Design review of the part built by this model. Coordinates are the model's own, in mm. Round coordinates to 2 decimals unless told otherwise and drop trailing zeros. Order: outer loops, then holes, each group sorted by start corner. A loop starts at its lowest first (then second) coordinate and runs counter-clockwise, first axis right, second up. Notation, with made-up numbers: (-6, 60) - (40, 60) arc R37 cw to (40, 96) - close; hole circle Ø3 at (65.5, -15.75). An arc over 180 degrees is marked (long way). Write item = value, one per line.
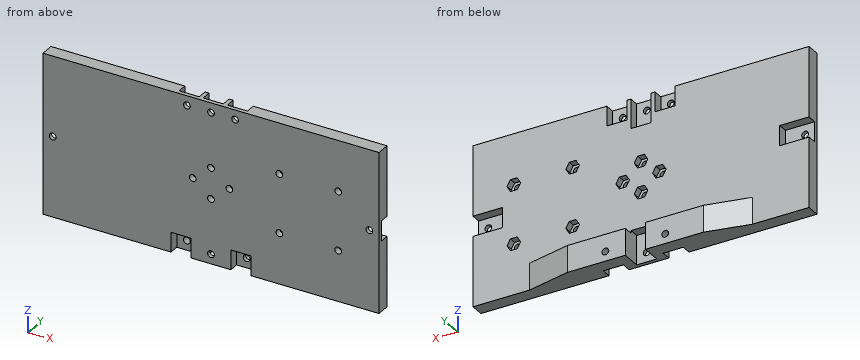
from build123d import *
from build123d.topology import SkipClean

# Parameters (mm, degrees)
SKETCH1_W           = 174.17
SKETCH1_H           = 83
BOSS_EXTRUDE1_DEPTH = 7
SKETCH2_R           = 1.75
CUT_EXTRUDE1_DEPTH  = 194.062655374
SKETCH3_R           = 1.75
CUT_EXTRUDE2_DEPTH  = 194.062655374
SKETCH4_W           = 15.4
SKETCH4_H           = 10.4
SKETCH4_W_2         = 10.4
SKETCH4_H_2         = 15.4
CUT_EXTRUDE3_DEPTH  = 5
SKETCH5_W           = 10.4
SKETCH5_H           = 10.4
CUT_EXTRUDE4_DEPTH  = 5
SKETCH6_R           = 1.75
CUT_EXTRUDE5_DEPTH  = 194.000489378
SKETCH12_R          = 1.75
CUT_EXTRUDE9_DEPTH  = 194.062655374
CUT_EXTRUDE6_DEPTH  = 3.64
SKETCH9_W           = 10.4
SKETCH9_H           = 10.4
CUT_EXTRUDE7_DEPTH  = 5
SKETCH10_R          = 1.75
CUT_EXTRUDE8_DEPTH  = 194.000489378
SKETCH13_W          = 20.6
SKETCH13_H          = 13.86
SKETCH13_R          = 1.75
BOSS_EXTRUDE2_DEPTH = 5
CHAMFER1_SIZE       = 7.094229205
CHAMFER1_SIZE_2     = 32
MIRROR1_START       = -76.250259333
MIRROR1_DEPTH       = 7.110259333
MIRROR1_START_2     = -83
MIRROR1_2_DEPTH     = 3.2499999
MIRROR1_START_3     = -79.7500001
MIRROR1_3_DEPTH     = 3.499740767
MIRROR1_START_4     = 7
MIRROR1_4_OUTLINE_R = 1.75
MIRROR1_4_DEPTH     = 5


with BuildPart() as part:
    # Sketch1 → Boss-Extrude1 (new body)
    with BuildSketch(Plane(origin=(0, 0, 0), x_dir=(1, 0, 0), z_dir=(0, 1, 0))):
        with Locations((87.085, 41.5)):
            Rectangle(SKETCH1_W, SKETCH1_H)
    extrude(amount=BOSS_EXTRUDE1_DEPTH)

    # Sketch2 → Cut-Extrude1 (cut, through all)
    with BuildSketch(Plane(origin=(0, 7, 0), x_dir=(1, 0, 0), z_dir=(0, 1, 0))):
        with Locations(Location((87.085, 49.5, 0), (0, 0, 270))):
            Circle(SKETCH2_R)
        with Locations(Location((77.585, 41.5, 0), (0, 0, 270))):
            Circle(SKETCH2_R)
        with Locations(Location((96.585, 41.5, 0), (0, 0, 270))):
            Circle(SKETCH2_R)
        with Locations(Location((87.085, 33.5, 0), (0, 0, 270))):
            Circle(SKETCH2_R)
    extrude(amount=-CUT_EXTRUDE1_DEPTH, mode=Mode.SUBTRACT)

    # Sketch3 → Cut-Extrude2 (cut, through all)
    with BuildSketch(Plane(origin=(0, 7, 0), x_dir=(1, 0, 0), z_dir=(0, 1, 0))):
        with Locations(Location((87.085, 78, 0), (0, 0, 270))):
            Circle(SKETCH3_R)
        with Locations(Location((5, 41.5, 0), (0, 0, 270))):
            Circle(SKETCH3_R)
        with Locations(Location((87.085, 5, 0), (0, 0, 270))):
            Circle(SKETCH3_R)
        with Locations(Location((169.17, 41.5, 0), (0, 0, 270))):
            Circle(SKETCH3_R)
    extrude(amount=-CUT_EXTRUDE2_DEPTH, mode=Mode.SUBTRACT)

    # Sketch4 → Cut-Extrude3 (cut)
    with BuildSketch(Plane(origin=(0, 7, 0), x_dir=(1, 0, 0), z_dir=(0, 1, 0))):
        with Locations((7.5, 41.5)):
            Rectangle(SKETCH4_W, SKETCH4_H)
        with Locations((87.085, 7.5)):
            Rectangle(SKETCH4_W_2, SKETCH4_H_2)
        with Locations((87.085, 75.5)):
            Rectangle(SKETCH4_W_2, SKETCH4_H_2)
        with Locations((166.67, 41.5)):
            Rectangle(SKETCH4_W, SKETCH4_H)
    extrude(amount=-CUT_EXTRUDE3_DEPTH, mode=Mode.SUBTRACT)

    # Sketch5 → Cut-Extrude4 (cut)
    with BuildSketch(Plane(origin=(0, 7, 0), x_dir=(1, 0, 0), z_dir=(0, 1, 0))):
        with Locations((74.585, 5)):
            Rectangle(SKETCH5_W, SKETCH5_H)
        with Locations((99.585, 5)):
            Rectangle(SKETCH5_W, SKETCH5_H)
    extrude(amount=-CUT_EXTRUDE4_DEPTH, mode=Mode.SUBTRACT)

    # Sketch6 → Cut-Extrude5 (cut, through all)
    with BuildSketch(Plane(origin=(0, 2, 0), x_dir=(1, 0, 0), z_dir=(0, 1, 0))):
        with Locations(Location((74.585, 5, 0), (0, 0, 270))):
            Circle(SKETCH6_R)
        with Locations(Location((99.585, 5, 0), (0, 0, 270))):
            Circle(SKETCH6_R)
    extrude(amount=-CUT_EXTRUDE5_DEPTH, mode=Mode.SUBTRACT)

    # Sketch12 → Cut-Extrude9 (cut, through all)
    with BuildSketch(Plane.XZ):
        with Locations(Location((122.51393219, -26.25, 0), (0, 0, 270))):
            Circle(SKETCH12_R)
        with Locations(Location((153.01393219, -26.25, 0), (0, 0, 270))):
            Circle(SKETCH12_R)
        with Locations(Location((122.51393219, -56.75, 0), (0, 0, 270))):
            Circle(SKETCH12_R)
        with Locations(Location((153.01393219, -56.75, 0), (0, 0, 270))):
            Circle(SKETCH12_R)
    extrude(amount=-CUT_EXTRUDE9_DEPTH, mode=Mode.SUBTRACT)

    # Sketch7 → Cut-Extrude6 (cut)
    with BuildSketch(Plane(origin=(0, 7, 0), x_dir=(1, 0, 0), z_dir=(0, 1, 0))):
        Polygon((75.824081679, 44.55), (79.345918321, 44.55), (81.106836642, 41.5), (79.345918321, 38.45), (75.824081679, 38.45), (74.063163358, 41.5), align=None)
        Polygon((85.324081679, 52.55), (88.845918321, 52.55), (90.606836642, 49.5), (88.845918321, 46.45), (85.324081679, 46.45), (83.563163358, 49.5), align=None)
        Polygon((100.106836642, 41.5), (98.345918321, 44.55), (94.824081679, 44.55), (93.063163358, 41.5), (94.824081679, 38.45), (98.345918321, 38.45), align=None)
        Polygon((83.563163358, 33.5), (85.324081679, 30.45), (88.845918321, 30.45), (90.606836642, 33.5), (88.845918321, 36.55), (85.324081679, 36.55), align=None)
        Polygon((120.753013869, 29.3), (124.274850511, 29.3), (126.035768832, 26.25), (124.274850511, 23.2), (120.753013869, 23.2), (118.992095548, 26.25), align=None)
        Polygon((151.253013869, 29.3), (154.774850511, 29.3), (156.535768832, 26.25), (154.774850511, 23.2), (151.253013869, 23.2), (149.492095548, 26.25), align=None)
        Polygon((151.253013869, 59.8), (154.774850511, 59.8), (156.535768832, 56.75), (154.774850511, 53.7), (151.253013869, 53.7), (149.492095548, 56.75), align=None)
        Polygon((120.753013869, 59.8), (124.274850511, 59.8), (126.035768832, 56.75), (124.274850511, 53.7), (120.753013869, 53.7), (118.992095548, 56.75), align=None)
    extrude(amount=-CUT_EXTRUDE6_DEPTH, mode=Mode.SUBTRACT)

    # Sketch9 → Cut-Extrude7 (cut)
    with BuildSketch(Plane.XZ):
        with Locations((71.585, -78)):
            Rectangle(SKETCH9_W, SKETCH9_H)
        with Locations((102.585, -78)):
            Rectangle(SKETCH9_W, SKETCH9_H)
    extrude(amount=-CUT_EXTRUDE7_DEPTH, mode=Mode.SUBTRACT)

    # Sketch10 → Cut-Extrude8 (cut, through all)
    with BuildSketch(Plane.XZ.offset(-5)):
        with Locations(Location((71.585, -78, 0), (0, 0, 270))):
            Circle(SKETCH10_R)
        with Locations(Location((102.585, -78, 0), (0, 0, 270))):
            Circle(SKETCH10_R)
    extrude(amount=-CUT_EXTRUDE8_DEPTH, mode=Mode.SUBTRACT)

    # Sketch13 → Boss-Extrude2 (add)
    with BuildSketch(Plane(origin=(0, 7, 0), x_dir=(1, 0, 0), z_dir=(0, 1, 0))):
        with Locations((71.585, 76.07)):
            Rectangle(SKETCH13_W, SKETCH13_H)
        with Locations(Location((71.585, 78, 0), (0, 0, 90))):
            Circle(SKETCH13_R, mode=Mode.SUBTRACT)
    extrude(amount=BOSS_EXTRUDE2_DEPTH)

    # Chamfer1
    # the kernel refuses this chamfer: 32, 7.094229205 mm, written as the material it adds along each edge
    with BuildSketch(Plane(origin=(61.285, 7, -83), x_dir=(0, 1, 0), z_dir=(0, 0, 1))) as chamfer1_piece_1_section:
        Polygon((CHAMFER1_SIZE, 0), (0, CHAMFER1_SIZE_2), (0, 0), align=None)
    chamfer1_piece_1 = extrude(amount=13.86, mode=Mode.PRIVATE)
    chamfer1_piece_1 = split(chamfer1_piece_1, bisect_by=Plane(origin=(61.285, 12, -83), z_dir=(0, -1, 0)), keep=Keep.TOP, mode=Mode.PRIVATE)
    add(chamfer1_piece_1)

    # Mirror1: read off the stored shape, not the designer's step
    # Mirror1 outline → Mirror1 (add)
    with BuildSketch(Plane.XY.offset(MIRROR1_START)):
        Polygon((92.285, 12), (92.285, 7), (144.885, 7), (122.331457482, 12), align=None)
    extrude(amount=MIRROR1_DEPTH)

    # Mirror1 2 outline → Mirror1 2 (add)
    with BuildSketch(Plane.XY.offset(MIRROR1_START_2)):
        Polygon((92.285, 12), (92.285, 7), (144.885, 7), (122.331457482, 12), align=None)
    extrude(amount=MIRROR1_2_DEPTH)

    # Mirror1 3 outline → Mirror1 3 (add)
    with BuildSketch(Plane.XY.offset(MIRROR1_START_3)):
        Polygon((92.285, 12), (92.285, 7), (144.885, 7), (122.331457482, 12), align=None)
    extrude(amount=MIRROR1_3_DEPTH)

    # Mirror1 4 outline → Mirror1 4 (cut)
    with SkipClean():  # the faces are left unmerged after this step: merging them gives an invalid solid
        with BuildSketch(Plane(origin=(0, 0, 0), x_dir=(1, 0, 0), z_dir=(0, 1, 0)).offset(MIRROR1_START_4)):
            with Locations((102.585, 78)):
                Circle(MIRROR1_4_OUTLINE_R)
        extrude(amount=MIRROR1_4_DEPTH, mode=Mode.SUBTRACT)
    add(part.part.scale(1), mode=Mode.REPLACE)  # the faces are merged on a copy


solid = part.part
Item 1: For line 1 along X through (y, z) = (1.05, -26.25); line 2 along Z through (x, y) = (164, 4); line 3 along X through (y, z) = (6.5, -43.5), list the stretches that pass through material, from the lowest coordinate up. Write a range as [from, to].
Data:
line_1 = [0, 120.76], [124.26, 151.26], [154.76, 174.17]
line_2 = [-83, -46.7], [-36.3, 0]
line_3 = [15.2, 75.22], [79.95, 94.22], [98.95, 158.97]
Item 2: Take a section at C-C, the plane x = 36. State the section outline as (y, z) points, and give its area (3 significant figures).
Data:
outline = (0, -83) - (8.49, -83) - (8.49, -69.14) - (7, -69.14) - (7, 0) - (0, 0) - close
area = 602 mm2
Item 3: Take a section at B-B, the plane z = -17. State the section outline as (x, y) points, and give its area (3 significant figures).
Data:
outline = (0, 0) - (174.17, 0) - (174.17, 7) - (0, 7) - close
area = 1,220 mm2
Item 4: Take a section at A-A, the plane x = 169.17. State the section outline as (y, z) points.
Data:
outline = (0, -83) - (7, -83) - (7, -46.7) - (2, -46.7) - (2, -43.25) - (0, -43.25) - close; (0, -39.75) - (2, -39.75) - (2, -36.3) - (7, -36.3) - (7, 0) - (0, 0) - close
Item 5: Insertion check: P1, Ø2.5, axis at x = 108, y = 9, coming from the +Z side; P2, Ø5.5, axis at x = 102.585, z = -78, coming from the -Y side; P3, Ø10, axis at x = 87.5, z = -30.5, coming from the +Y side. Each pin has a flat end and moves straight along its axis. Give the tip position at first contact, or say it passes through.
Data:
P1 = -69.14
P2 = 5
P3 = 7
